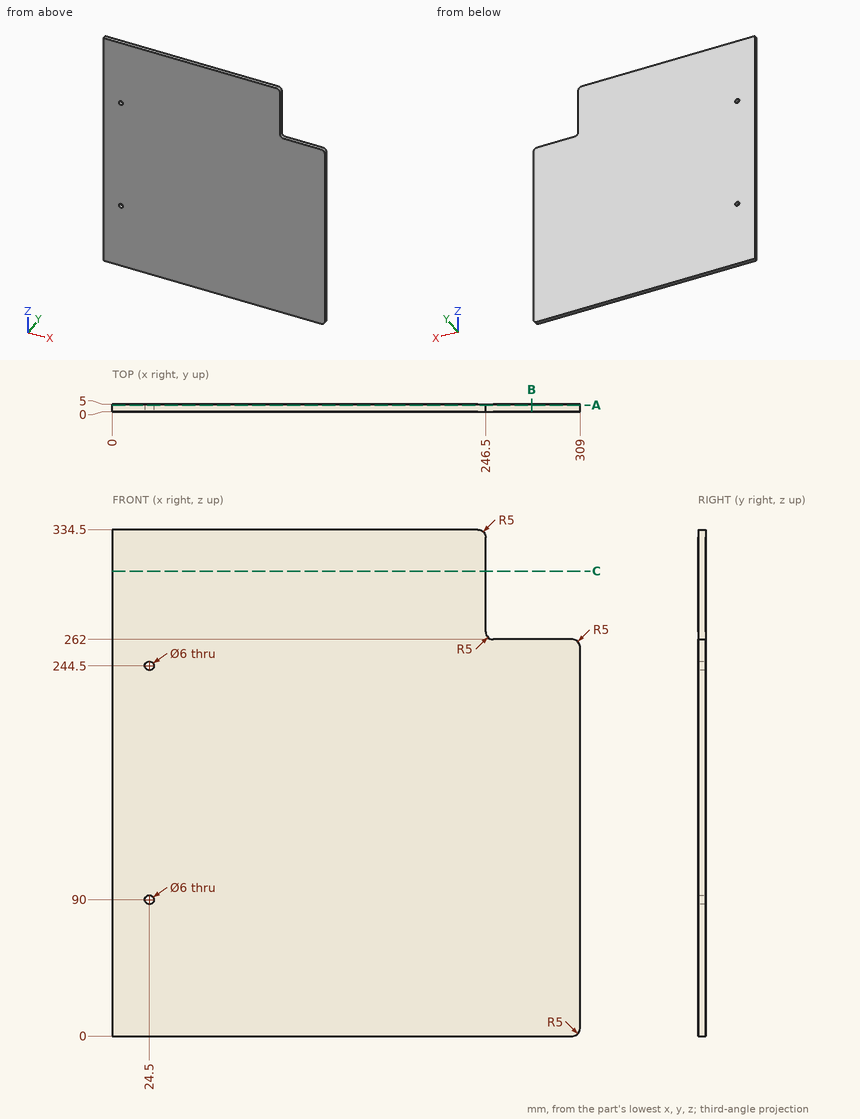
Geometry check sheet. Reference: drawing and pictorial views, mm from the part's lowest x, y, z. Coordinates: 2 decimals unless noted, no trailing zeros. Write each loop counter-clockwise with the first axis right and the second up, starting at its lowest first coordinate (ties: lowest second). Pieces come first, ordered by that corner, then holes. Notation, with made-up numbers: (-39.75, 13) -> (15.25, 13) arc R21 cw to (15.25, 33) -> close; hole circle Ø5 at (61, 24.25). An arc over 180 degrees is marked (long way). One line per question, with ' | ' between items.
1. Thickness scan on probe 1 along X at (y, z) = (1.05, 244.5); probe 2 along X at (y, z) = (1.8, 281); probe 3 along Z at (x, y) = (252.5, 0.6). Record the ranges inside material, lowest first. Write a range as from..to.
Answers:
probe 1: x = 0..21.5, 27.5..309 | probe 2: x = 0..246.5 | probe 3: z = 0..262
2. Cross-section at B-B on x = 277. Record the cut outline in (y, z).
Answers:
outline: (0, 0) -> (5, 0) -> (5, 262) -> (0, 262) -> close
3. Cross-section at A-A on y = 4.25. Record the cut outline in (x, z), and give its area (3 significant figures).
Answers:
outline: (0, 0) -> (304, 0) arc R5 ccw to (309, 5) -> (309, 257) arc R5 ccw to (304, 262) -> (251.5, 262) arc R5 cw to (246.5, 267) -> (246.5, 329.5) arc R5 ccw to (241.5, 334.5) -> (0, 334.5) -> close; hole circle Ø6 at (24.5, 90); hole circle Ø6 at (24.5, 244.5) | area: 98,800 mm²
4. Cross-section at C-C on z = 307. Record the cut outline in (x, y), and give its area (3 significant figures).
Answers:
outline: (0, 0) -> (246.5, 0) -> (246.5, 5) -> (0, 5) -> close | area: 1,230 mm²
5. Depth check by flat-ended pin: pin 1 Ø2 at (x, z) = (195, 295) entering from -Y; pin 2 Ø2.5 at (x, y) = (265, 3) entering from +Z. Enter the tip coordinate at first touch or a pass-through.
Answers:
pin 1: stops at y = 0 | pin 2: stops at z = 262
